Geometry check sheet. Reference: the model listing, model coordinates, mm. A direction names the side the tool comes from. Give positions to 0.01 mm unless a question says otherwise; leave off trailing zeros. Order: outer loops, then holes, each group sorted by start corner. A loop starts at its lowest first (then second) coordinate and runs counter-clockwise, first axis right, second up. Notation, with made-up numbers: M -39,57.5 L -10,57.5 A11 ccw -10,75.5 Z; hole C 88,-20 d1. An arc over 180 degrees is marked long. Put each result on its own line as item: value. Start each with the question number.
Q1. Go/stop test with flat-tipped pins: pin 1 (2 mm diameter, centred on x = -13, y = 13, fed in from +Z); pin 2 (1.6 mm diameter, centred on y = 14.5, z = 1, fed in from -X); pin 3 (0.8 mm diameter, centred on y = -3.5, z = 0.5, fed in from +X); pin 4 (3 mm diameter, centred on y = 9.5, z = 5.5, fed in from +X). Record where each tip stops, or that it passes through.
Q2. Material ranges on L1, parallel to X at y = 1.15, z = 7.75; L2, parallel to X at y = 7.25, z = 10.25; L3, parallel to X at y = -3.5, z = 7.75, recorded low to high.
Q3. Section check C-C on x = 12.5. Record the cut outline in (y, z), then the cut area to 4 significant figures.
Q4. Section check D-D on y = 2.25. Record the cut outline in (x, z).
Q5. Mould release check, pull along Z, two halves, no side actions. Record for faces 1 (the flat face through (-14, 5.495, 6)), 2 (the flat face through (-14, 8, 11.5)), 3 (the cylindrical face through (-13.1, -1.3, 8.5)): +Z half, -Z half, draft (parallel to the pull), parting line (faces both ways), or undercut.
Q6. Section check A-A on z = 2.25. Record the cut outline in (x, y).
Q7. Section check B-B on y = -3. Record the cut outline in (x, z), then the cut area to 3 significant figures.
Q8. Access from +Z, -Z, +X, -X, +Y, -Y to the whole of each face (thin tool, end or side, straight path). Record for faces 4 (the flat face through (10.937, 15, 1)), 5 (the flat face through (13, 5.495, 6)), 6 (the flat face through (10.937, 9, 6)), 7 (the flat face through (-11.663, 15, 1)), 8 (the flat face through (3.157, -3, 1)).
```python
from build123d import *

# Parameters (mm, degrees)
SKETCH_1_W          = 32.4
SKETCH_1_H          = 30
EXTRUDE_1_DEPTH     = 1.5
SKETCH_2_W          = 4.9
SKETCH_2_H          = 8.52
EXTRUDE_2_DEPTH     = 10
CUT_EXTRUDE_1_DEPTH = 11.5
SKETCH_4_R          = 1.3
CUT_EXTRUDE_2_DEPTH = 31.5


with BuildPart() as part:
    # 草图1 → 凸台-拉伸1 (new body)
    with BuildSketch(Plane.XY):
        with Locations((-0.362675268, 2.133428793)):
            Rectangle(SKETCH_1_W, SKETCH_1_H)
    extrude(amount=EXTRUDE_1_DEPTH)

    # 草图2 → 凸台-拉伸2 (add)
    with BuildSketch(Plane.XY.offset(1.5)):
        with Locations((-14.112675268, -1.225199495)):
            Rectangle(SKETCH_2_W, SKETCH_2_H)
        Polygon((-16.562675268, 5.494800505), (-11.662675268, 5.494800505), (-11.662675268, 12.70812694), (-16.562675268, 7.80812694), align=None)
        Polygon((10.937324732, 5.494800505), (10.937324732, 12.70812694), (15.837324732, 7.80812694), (15.837324732, 5.494800505), align=None)
        Polygon((10.937324732, 3.034800505), (15.837324732, 3.034800505), (15.837324732, 0), (10.937324732, -1.245199495), align=None)
    extrude(amount=EXTRUDE_2_DEPTH)

    # 草图3 → 切除-拉伸1 (cut)
    with BuildSketch(Plane.XY.offset(1.5)):
        Polygon((-16.562675268, 7.80812694), (-11.662675268, 12.70812694), (-11.662675268, 17.133428793), (-16.562675268, 17.133428793), align=None)
        Polygon((15.837324732, 7.80812694), (10.937324732, 12.70812694), (10.937324732, 17.133428793), (15.837324732, 17.133428793), align=None)
        Polygon((-16.562675268, -12.866571207), (-16.562675268, -8.702000753), (-16.562675268, -5.485199495), (3.157324732, -5.485199495), (3.157324732, -1.245199495), (10.937324732, -1.245199495), (15.837324732, 0), (15.837324732, -12.866571207), align=None)
    extrude(amount=-CUT_EXTRUDE_1_DEPTH, mode=Mode.SUBTRACT)

    # 草图4 → 切除-拉伸2 (cut)
    with BuildSketch(Plane.XZ.offset(5.485199495)):
        with Locations(Location((-14.162675268, 7.75, 0), (0, 0, 180))):
            Circle(SKETCH_4_R)
        with Locations(Location((13.437324732, 7.75, 0), (0, 0, 270))):
            Circle(SKETCH_4_R)
    extrude(amount=-CUT_EXTRUDE_2_DEPTH, mode=Mode.SUBTRACT)


solid = part.part
```
Results found:
1. pin 1: passes through
1. pin 2: stops at x = -11.66
1. pin 3: stops at x = 3.16
1. pin 4: stops at x = 15.65
2. L1: x = -16.56 to -15.46, -12.86 to -11.66, 10.94 to 12.14, 14.74 to 15.84
2. L2: x = -16.56 to -11.66, 10.94 to 15.84
2. L3: x = -16.56 to -15.46, -12.86 to -11.66
3. outline: M -0.85,0 L 11.15,0 L 11.15,6.85 L 5.49,6.85 L 5.49,1.5 L 3.03,1.5 L 3.03,6.85 L -0.85,6.85 Z; M -0.85,8.65 L 3.03,8.65 L 3.03,11.5 L -0.85,11.5 Z; M 5.49,8.65 L 11.15,8.65 L 11.15,11.5 L 5.49,11.5 Z
3. area: 96.15 mm^2
4. outline: M -16.56,0 L 15.84,0 L 15.84,11.5 L 10.94,11.5 L 10.94,1.5 L -11.66,1.5 L -11.66,11.5 L -16.56,11.5 Z; hole C -14.16,7.75 d2.6; hole C 13.44,7.75 d2.6
5. face 1: draft
5. face 2: +Z half
5. face 3: undercut
6. outline: M -16.56,-5.49 L -11.66,-5.49 L -11.66,3.03 L -16.56,3.03 Z; M -16.56,5.49 L -11.66,5.49 L -11.66,12.71 L -16.56,7.81 Z; M 10.94,-1.25 L 15.84,0 L 15.84,3.03 L 10.94,3.03 Z; M 10.94,5.49 L 15.84,5.49 L 15.84,7.81 L 10.94,12.71 Z
7. outline: M -16.56,0 L 3.16,0 L 3.16,1.5 L -11.66,1.5 L -11.66,11.5 L -16.56,11.5 Z; hole C -14.16,7.75 d2.6
7. area: 73.3 mm^2
8. face 4: +Z, -Z, +X, +Y
8. face 5: +Z, +X, -X
8. face 6: +Z, +Y, -Y
8. face 7: +Z, -Z, -X, +Y
8. face 8: +Z, -Z, +X, -Y
